Part model, mm, in its own coordinate system. A direction names the side the tool comes from. Coordinates: 2 decimals unless noted, no trailing zeros. Order: outer loops, then holes, each group sorted by start corner. A loop starts at its lowest first (then second) coordinate and runs counter-clockwise, first axis right, second up.
1) Wall check: L1, parallel to X at y = 0.5, z = -17.8; L2, parallel to Y at x = 7, z = -1.5; L3, parallel to Y at x = 16.5, z = -14. Give the ranges that are in metal, low to high.
2) Mould opens along Z. For faces 1 (the flat face through (0, 3, 4.872)), 2 (the flat face through (-6.92, 2.19, 4.02)), 3 (the flat face through (8.1, 2.857, -4.715)), 4 (the flat face through (0, 26.6, 0)) say: +Z half, -Z half, draft (parallel to the pull), parting line (faces both ways), or undercut.
3) Pin check, flat tips, straight feed: pin 1 Ø5 at (y, z) = (17, 12) entering from -X; pin 2 Ø5 at (y, z) = (11, 11) entering from -X; pin 3 Ø0.8 at (y, z) = (3, 6.5) entering from -X. Stop position of each tip, or through.
4) Tool access for faces 5 (the flat face through (1.2, 2, -7)), 6 (the flat face through (13.1, 3, 0)), 7 (the flat face through (-5.804, 2.192, 4.737)): list every direction of +Z, -Z, +X, -X, +Y, -Y with a clear straight run to the whole face (end or side of a thin tool).
5) Cut at C-C (y = 15.5). List the corners of the cut face in (x, z), and give its area (3 significant figures).
6) Cut at B-B (y = 18.75). List the corners of the cut face in (x, z).
7) Cut at A-A (z = -17.8). List the corners of the cut face in (x, y), and give its area (3 significant figures).
```python
from build123d import *

# Parameters (mm, degrees)
SKETCH1_W           = 36.2
SKETCH1_H           = 41.3
SKETCH1_R           = 1.6
BOSS_EXTRUDE1_DEPTH = 1.6
SKETCH2_W           = 5.2
SKETCH2_H           = 6.5
BOSS_EXTRUDE2_DEPTH = 2.95
SKETCH3_W           = 4.7
SKETCH3_H           = 4.5
BOSS_EXTRUDE3_DEPTH = 2.55
SKETCH4_W           = 2.4
SKETCH4_H           = 1.2
BOSS_EXTRUDE4_DEPTH = 1.2
SKETCH5_R           = 12.1
SKETCH5_R_2         = 12
CUT_EXTRUDE1_DEPTH  = 0.05
SKETCH6_R           = 0.375
CUT_EXTRUDE2_DEPTH  = 28.825752461
CIRPATTERN2_COUNT   = 3
CUT_EXTRUDE3_DEPTH  = 0.1


with BuildPart() as part:
    # Sketch1 → Boss-Extrude1 (new body)
    with BuildSketch(Plane(origin=(0, 0, 0), x_dir=(1, 0, 0), z_dir=(0, 1, 0))):
        Rectangle(SKETCH1_W, SKETCH1_H)
        with Locations(Location((-10.15, 17.8, 0), (0, 0, 270))):
            Circle(SKETCH1_R, mode=Mode.SUBTRACT)
        with Locations(Location((10.15, 17.8, 0), (0, 0, 270))):
            Circle(SKETCH1_R, mode=Mode.SUBTRACT)
        with Locations(Location((-10.15, -17.8, 0), (0, 0, 270))):
            Circle(SKETCH1_R, mode=Mode.SUBTRACT)
        with Locations(Location((10.15, -17.8, 0), (0, 0, 270))):
            Circle(SKETCH1_R, mode=Mode.SUBTRACT)
    extrude(amount=BOSS_EXTRUDE1_DEPTH)

    # Sketch2 → Boss-Extrude2 (add)
    with BuildSketch(Plane(origin=(0, 1.6, 0), x_dir=(1, 0, 0), z_dir=(0, 1, 0))):
        with Locations((-15.7, 0)):
            Rectangle(SKETCH2_W, SKETCH2_H)
        with Locations((15.7, 0)):
            Rectangle(SKETCH2_W, SKETCH2_H)
    extrude(amount=BOSS_EXTRUDE2_DEPTH)

    # Sketch3 → Boss-Extrude3 (add)
    with BuildSketch(Plane(origin=(0, 1.6, 0), x_dir=(1, 0, 0), z_dir=(0, 1, 0))):
        Polygon((-6.941670728, 6.721321728), (-3.04455641, 4.471321728), (-5.39455641, 0.401002331), (-9.291670728, 2.651002331), align=None)
        Polygon((3.04455641, 4.471321728), (6.941670728, 6.721321728), (9.291670728, 2.651002331), (5.39455641, 0.401002331), align=None)
        with Locations((0, -7.122324059)):
            Rectangle(SKETCH3_W, SKETCH3_H)
    extrude(amount=BOSS_EXTRUDE3_DEPTH)

    # Sketch4 → Boss-Extrude4 (add)
    with BuildSketch(Plane(origin=(0, 1.6, 0), x_dir=(1, 0, 0), z_dir=(0, 1, 0))):
        with Locations((0, 7.403377608)):
            Rectangle(SKETCH4_W, SKETCH4_H)
        Polygon((6.49189784, -2.362458319), (5.29189784, -4.440919288), (6.331128324, -5.040919288), (7.531128324, -2.962458319), align=None)
        Polygon((-6.49189784, -2.362458319), (-5.29189784, -4.440919288), (-6.331128324, -5.040919288), (-7.531128324, -2.962458319), align=None)
    extrude(amount=BOSS_EXTRUDE4_DEPTH)

    # Sketch5 → Cut-Extrude1 (cut)
    with BuildSketch(Plane(origin=(0, 1.6, 0), x_dir=(1, 0, 0), z_dir=(0, 1, 0))):
        with Locations(Location((0, 0, 0), (0, 0, 270))):
            Circle(SKETCH5_R)
        with Locations(Location((0, 0, 0), (0, 0, 270))):
            Circle(SKETCH5_R_2, mode=Mode.SUBTRACT)
    extrude(amount=-CUT_EXTRUDE1_DEPTH, mode=Mode.SUBTRACT)

    # Sketch6 → Cut-Extrude2 (cut, through all)
    with BuildSketch(Plane(origin=(0, 3.6, 0), x_dir=(1, 0, 0), z_dir=(0, 1, 0))):
        with Locations(Location((-6.674097159, 3.853291792, 0), (0, 0, 270))):
            Circle(SKETCH6_R)
        with Locations(Location((6.674097159, 3.853291792, 0), (0, 0, 270))):
            Circle(SKETCH6_R)
        with Locations(Location((0, -7.706583583, 0), (0, 0, 270))):
            Circle(SKETCH6_R)
    extrude(amount=CUT_EXTRUDE2_DEPTH, mode=Mode.SUBTRACT)

    # Sketch7 → Revolve3 (revolve)
    with BuildSketch(Plane(origin=(0, 0, 0), x_dir=(0, 0, -1), z_dir=(1, 0, 0)), mode=Mode.PRIVATE) as revolve3_sk:
        Polygon((1.967510892, 26.6), (-7.706583583, 26.6), (-7.706583583, 3.6), (-7.331583583, 3.6), (-7.331583583, 4.15), align=None)
    revolve3 = revolve(revolve3_sk.sketch.rotate(Axis((0, 26.6, 7.706583583), (0, -1, 0)), 180), axis=Axis((0, 26.6, 7.706583583), (0, -1, 0)))

    # CirPattern2: Revolve3 ×3 about axis
    cirpattern2_axis = Axis((0, 0, 0), (0, 1, 0))
    for i in range(1, CIRPATTERN2_COUNT):
        add(revolve3.rotate(cirpattern2_axis, i * 360 / CIRPATTERN2_COUNT))

    # Sketch8 → Cut-Extrude3 (cut)
    with BuildSketch(Plane(origin=(0, 26.6, 0), x_dir=(1, 0, 0), z_dir=(0, 1, 0))):
        with BuildLine():
            Line((-9.49791005, -5.399501553), (-9.425060538, -5.52568061))
            ThreePointArc((-9.425060538, -5.52568061), (-4.415728318, -5.656318768), (0, -3.287390943))
            ThreePointArc((0, -3.287390943), (4.415728318, -5.656318768), (9.425060538, -5.52568061))
            Line((9.425060538, -5.52568061), (9.49791005, -5.399501553))
            ThreePointArc((9.49791005, -5.399501553), (7.106379904, -0.995973516), (2.846964069, 1.643695472))
            ThreePointArc((2.846964069, 1.643695472), (2.690651586, 6.652292283), (0.072849512, 10.925182163))
            Line((0.072849512, 10.925182163), (-0.072849512, 10.925182163))
            ThreePointArc((-0.072849512, 10.925182163), (-2.690651586, 6.652292283), (-2.846964069, 1.643695472))
            ThreePointArc((-2.846964069, 1.643695472), (-7.106379904, -0.995973516), (-9.49791005, -5.399501553))
        make_face()
        with BuildLine():
            ThreePointArc((0, -3.011088161), (1.617311874, -0.933755446), (2.60767884, 1.50554408))
            ThreePointArc((2.60767884, 1.50554408), (0, 1.867510892), (-2.60767884, 1.50554408))
            ThreePointArc((-2.60767884, 1.50554408), (-1.617311874, -0.933755446), (0, -3.011088161))
        make_face(mode=Mode.SUBTRACT)
        with BuildLine():
            ThreePointArc((0, 10.717671744), (-2.510270593, 6.557117602), (-2.654727509, 1.700081323))
            ThreePointArc((-2.654727509, 1.700081323), (0, 2.067510892), (2.654727509, 1.700081323))
            ThreePointArc((2.654727509, 1.700081323), (2.510270593, 6.557117602), (0, 10.717671744))
        make_face(mode=Mode.SUBTRACT)
        with BuildLine():
            ThreePointArc((-9.281776, -5.358835872), (-4.423495123, -5.452516905), (-0.14494986, -3.149102125))
            ThreePointArc((-0.14494986, -3.149102125), (-1.790516955, -1.033755446), (-2.799677369, 1.449020802))
            ThreePointArc((-2.799677369, 1.449020802), (-6.933765715, -1.104600697), (-9.281776, -5.358835872))
        make_face(mode=Mode.SUBTRACT)
        with BuildLine():
            ThreePointArc((9.281776, -5.358835872), (6.933765715, -1.104600697), (2.799677369, 1.449020802))
            ThreePointArc((2.799677369, 1.449020802), (1.790516955, -1.033755446), (0.14494986, -3.149102125))
            ThreePointArc((0.14494986, -3.149102125), (4.423495123, -5.452516905), (9.281776, -5.358835872))
        make_face(mode=Mode.SUBTRACT)
    extrude(amount=-CUT_EXTRUDE3_DEPTH, mode=Mode.SUBTRACT)


solid = part.part
```
Geometry check:
1. L1: x = -18.1 to -11.75, -8.55 to 8.55, 11.75 to 18.1
1. L2: y = 0 to 4.15, 8.98 to 26.6
1. L3: y = 0 to 1.6
2. face 1: undercut
2. face 2: +Z half
2. face 3: -Z half
2. face 4: draft
3. pin 1: stops at x = -5.91
3. pin 2: stops at x = -3.64
3. pin 3: stops at x = -2.35
4. face 5: -Z, +X
4. face 6: +Z, -Z
4. face 7: +Z
5. outline: circle Ø10.15 at (-6.67, -3.85); circle Ø10.15 at (0, 7.71); circle Ø10.15 at (6.67, -3.85)
5. area: 243 mm2
6. outline: circle Ø12.85 at (-6.67, -3.85); circle Ø12.85 at (0, 7.71); circle Ø12.85 at (6.67, -3.85)
7. outline: (-18.1, 0) - (-11.75, 0) - (-11.75, 1.6) - (-18.1, 1.6) - close; (-8.55, 0) - (8.55, 0) - (8.55, 1.6) - (-8.55, 1.6) - close; (11.75, 0) - (18.1, 0) - (18.1, 1.6) - (11.75, 1.6) - close
7. area: 47.7 mm2
